```python
from build123d import *

# Parameters (mm, degrees)
F1_DEPTH = 10.87167
F2_W     = 20.7378324121
F2_H     = 41.1411811365
F3_DEPTH = 9.78587
F4_W     = 8.6351763457
F4_H     = 6.0070783366
F5_DEPTH = 63.13654


with BuildPart() as f1:
    # F0 (on Top) → F1 (new body)
    with BuildSketch(Plane.XY):
        with BuildLine():
            ThreePointArc((-19.6146064737, 24.572059019), (-7.0926943283, 34.0930740127), (-19.6146064737, 43.6140890064))
            ThreePointArc((-19.6146064737, 43.6140890064), (-30.5177033911, 45.7644046028), (-41.4208003086, 43.6140890064))
            ThreePointArc((-41.4208003086, 43.6140890064), (-53.942712454, 34.0930740127), (-41.4208003086, 24.572059019))
            Line((-41.4208003086, 24.572059019), (-42.3597145092, 21.8851334871))
            ThreePointArc((-42.3597145092, 21.8851334871), (-47.713167553, 13.3357192606), (-46.4203947683, 3.3316859921))
            ThreePointArc((-46.4203947683, 3.3316859921), (-39.8100362087, -4.6984516114), (-30.8246676488, 0.5401648148))
            ThreePointArc((-30.8246676488, 0.5401648148), (-22.0252975249, -4.6761652077), (-15.660289069, 3.3316859921))
            ThreePointArc((-15.660289069, 3.3316859921), (-13.9296875224, 13.1566111484), (-18.7605294597, 21.8851334871))
            Line((-18.7605294597, 21.8851334871), (-19.6146064737, 24.572059019))
        make_face()
        with BuildLine():
            ThreePointArc((-30.7483132929, 5.6346026249), (-30.371478369, 3.0811636063), (-30.8246676488, 0.5401648148))
            ThreePointArc((-30.8246676488, 0.5401648148), (-31.2152322971, 3.0938096117), (-30.7483132929, 5.6346026249))
        make_face(mode=Mode.SUBTRACT)
        with BuildLine():
            ThreePointArc((-30.7483132929, 5.6346026249), (-31.2152322971, 3.0938096117), (-30.8246676488, 0.5401648148))
            ThreePointArc((-30.8246676488, 0.5401648148), (-30.371478369, 3.0811636063), (-30.7483132929, 5.6346026249))
        make_face()
    extrude(amount=F1_DEPTH)

    # F2 (on Top) → F3 (cut)
    with BuildSketch(Plane.XY):
        with Locations((-30.6165078655, 22.0384193235)):
            Rectangle(F2_W, F2_H)
    extrude(amount=F3_DEPTH, mode=Mode.SUBTRACT)

    # F4 (on Front) → F5 (cut)
    with BuildSketch(Plane.XZ):
        with Locations((-22.1452759579, 4.781266558)):
            Rectangle(F4_W, F4_H)
    extrude(amount=-F5_DEPTH, mode=Mode.SUBTRACT)


solid = f1.part
```
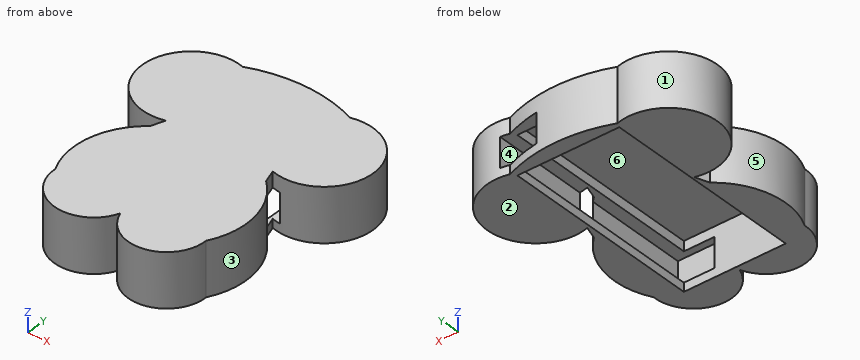
Check sheet for the modelled part. Datum: model origin and axes. Units: mm. Face numbers are marked on the shaded views. A direction names the side the tool comes from. Round coordinates to 2 decimals unless told otherwise and drop trailing zeros. Order: outer loops, then holes, each group sorted by start corner. A loop starts at its lowest first (then second) coordinate and runs counter-clockwise, first axis right, second up.
1) Section check C-C (y = 38.5). Record the boundary of the cut face in (x, z).
2) Section check B-B (x = -23.5). Record the boundary of the cut face in (y, z), and give its area (3 significant figures).
3) Section check D-D (x = -36). Record the boundary of the cut face in (y, z), and give its area (3 significant figures).
4) Scan lines: line 1 (X direction, y = 3, z = 4); line 2 (X direction, y = 3, z = 9.75); line 3 (Z direction, x = -24, y = 1). Record each from-to range of solid material in increasing order.
5) Mould release check, pull along X, two halves, no side actions. Record for the marked faces 1, 2 and 3: +X half, -X half, draft (parallel to the pull), parting line (faces both ways), or undercut.
6) Go/stop test with flat-tipped pins: pin 1 Ø5 at (x, z) = (-27.5, 6) entering from -Y; pin 2 Ø2 at (y, z) = (3, 2.5) entering from +X; pin 3 Ø5 at (x, z) = (-30, 2) entering from -Y. Record where each tip stops, or that it passes through.
7) Tool access check on the marked faces 4, 5 and 6. Record the directions out of +Z, -Z, +X, -X, +Y, -Y that give a thin tool (end or side, any length) a straight path to the whole face; none if there is none.
8) Section check A-A (z = 7). Record the boundary of the cut face in (x, y).
Result:
1. outline: (-52.91, 0) - (-40.99, 0) - (-40.99, 9.79) - (-20.25, 9.79) - (-20.25, 7.78) - (-17.83, 7.78) - (-17.83, 1.78) - (-20.25, 1.78) - (-20.25, 0) - (-8.13, 0) - (-8.13, 10.87) - (-52.91, 10.87) - close
2. outline: (-4.8, 0) - (1.47, 0) - (1.47, 1.78) - (0, 1.78) - (0, 7.78) - (1.47, 7.78) - (1.47, 9.79) - (42.61, 9.79) - (42.61, 7.78) - (44.89, 7.78) - (44.89, 10.87) - (-4.8, 10.87) - close; (42.61, 0) - (44.89, 0) - (44.89, 1.78) - (42.61, 1.78) - close
2. area: 115 mm2
3. outline: (-4.46, 0) - (1.47, 0) - (1.47, 9.79) - (42.61, 9.79) - (42.61, 0) - (45.24, 0) - (45.24, 10.87) - (-4.46, 10.87) - close
3. area: 138 mm2
4. line 1: x = -46.42 to -40.99, -17.83 to -15.65
4. line 2: x = -46.42 to -40.99, -20.25 to -15.65
4. line 3: z = 0 to 1.78, 7.78 to 10.87
5. face 1: undercut
5. face 2: draft
5. face 3: +X half
6. pin 1: stops at y = -4.65
6. pin 2: stops at x = -15.3
6. pin 3: stops at y = -3.66
7. face 4: +Y
7. face 5: +Z, -Z, -X
7. face 6: -Z
8. outline: (-46.42, 3.33) arc R8.03 ccw to (-30.82, 0.54) arc R7.78 ccw to (-15.66, 3.33) arc R14.96 ccw to (-17.83, 20.98) - (-17.83, 0) - (-26.46, 0) - (-26.46, 1.47) - (-40.99, 1.47) - (-40.99, 42.61) - (-26.46, 42.61) - (-26.46, 45.48) arc R28.72 ccw to (-41.42, 43.61) arc R9.88 ccw (long way) to (-41.42, 24.57) - (-42.36, 21.89) arc R14.96 ccw to start; (-17.83, 24.25) arc R9.88 ccw (long way) to (-17.83, 43.94) - close
